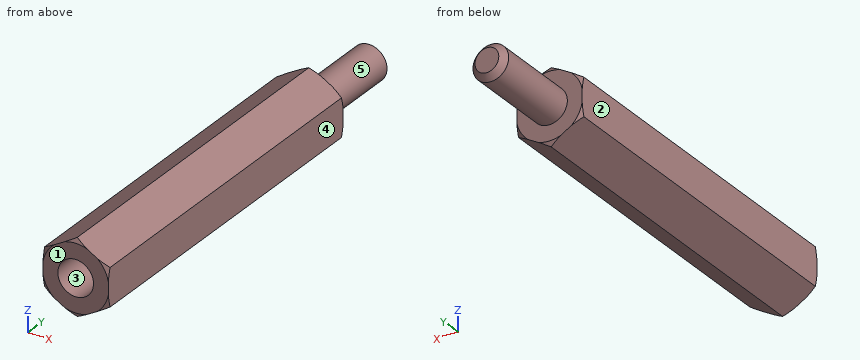
from build123d import *

# Parameters (mm, degrees)
SKETCH_1_R          = 1.5
EXTRUDE_1_DEPTH     = 30
SKETCH_3_R          = 1.5
EXTRUDE_2_DEPTH     = 8
CHAMFER_1_SIZE      = 0.5
SKETCH_1_3_R        = 1.5
CUT_EXTRUDE_1_DEPTH = 8


with BuildPart() as part:
    # Sketch 1 → Extrude 1 (new body)
    # profile 1 of 2: a face of its own
    with BuildSketch(Plane(origin=(0, 0, 0), x_dir=(1, 0, 0), z_dir=(0, 1, 0))):
        Polygon((2.75, -1.58771324), (2.75, 1.58771324), (0, 3.175426481), (-2.75, 1.58771324), (-2.75, -1.58771324), (0, -3.175426481), align=None)
        Circle(SKETCH_1_R, mode=Mode.SUBTRACT)
    # profile 2 of 2: a face of its own
    with BuildSketch(Plane(origin=(0, 0, 0), x_dir=(1, 0, 0), z_dir=(0, 1, 0))):
        Circle(SKETCH_1_R)
    extrude(amount=EXTRUDE_1_DEPTH)

    # Sketch 2 → Cut-Revolve 1 (revolve, cut)
    with BuildSketch(Plane(origin=(0, 0, 0), x_dir=(0, 0, -1), z_dir=(1, 0, 0))):
        Polygon((-26.160719749, 13.487317835), (-26.160719749, 0), (-2.8, 0), align=None)
        Polygon((-26.160719749, 30), (-26.160719749, 16.512682165), (-2.8, 30), align=None)
    revolve(axis=Axis((0, 30, 0), (0, -1, 0)), mode=Mode.SUBTRACT)

    # Sketch 3 → Extrude 2 (add)
    with BuildSketch(Plane(origin=(0, 30, 0), x_dir=(1, 0, 0), z_dir=(0, 1, 0))):
        with Locations(Location((0, 0, 0), (0, 0, 270))):
            Circle(SKETCH_3_R)
    extrude(amount=EXTRUDE_2_DEPTH)

    # Chamfer 1
    chamfer_1_edges = [part.edges().sort_by_distance(p)[0] for p in [
        (0, 38, -1.5),
    ]]
    chamfer(chamfer_1_edges, length=CHAMFER_1_SIZE)

    # Sketch 1_3 → Cut-Extrude 1 (cut)
    with BuildSketch(Plane(origin=(0, 0, 0), x_dir=(1, 0, 0), z_dir=(0, 1, 0))):
        with Locations(Location((0, 0, 0), (0, 0, 270))):
            Circle(SKETCH_1_3_R)
    extrude(amount=CUT_EXTRUDE_1_DEPTH, mode=Mode.SUBTRACT)


solid = part.part
Work out the finished part from the listing and answer in its coordinate system (mm). Face numbers are marked on the shaded views. A direction names the side the tool comes from. Give positions to 0.01 mm unless a question says otherwise; leave off trailing zeros. Order: outer loops, then holes, each group sorted by start corner. A loop starts at its lowest first (then second) coordinate and runs counter-clockwise, first axis right, second up. Notation, with made-up numbers: (63.25, -27) -> (67.25, -27) arc R18 cw to (67.25, -13) -> close; hole circle Ø7 at (39.25, -13). An arc over 180 degrees is marked (long way). Answer as a JSON object with one key per item and string values. Group by question number.
1. Consider line 1 along X through (y, z) = (2.25, 0); line 2 along Y through (x, z) = (-0.65, 0); line 3 along Y through (x, z) = (-1.9, 1.75). Determine where each line is inside the solid, lowest interval first. Write a range as [from, to].
2. Section A-A on y = 3 is taken. Determine the outline of the cut face in (x, z), plus the area to 3 significant figures.
3. Section C-C on y = 12 is taken. Determine the outline of the cut face in (x, z).
4. A tool of negligible diameter and unlimited length cuts with its end or side. For the marked faces 4 and 5, from which of +Z, -Z, +X, -X, +Y, -Y can it reach the whole face along a straight path? Write none if from no direction.
5. Flat-ended cylindrical pins translate along their axes: pin 1 Ø1 at (y, z) = (32, 1.5) entering from +X; pin 2 Ø1 at (x, y) = (-1, 14.5) entering from +Z; pin 3 Ø1 at (x, z) = (2, 1) entering from +Y. Find the tip coordinate at first contact, or state that the pin passes through.
6. Section D-D on y = 35 is taken. Determine the outline of the cut face in (x, z), plus the area to 3 significant figures.
7. Section B-B on z = 0 is taken. Determine the outline of the cut face in (x, y), plus the area to 3 significant figures.
8. The mould has two halves that part along X. Classify the marked faces 1, 2 and 3: released by +X, released by -X, zero draft, split by the parting line, or undercut.
Result sheet:
{
 "1": {"line 1": "x = [-2.75, -1.5], [1.5, 2.75]", "line 2": "y = [8, 38]", "line 3": "y = [0, 30]"},
 "2": {"outline": "(-2.75, -1.59) -> (0, -3.18) -> (2.75, -1.59) -> (2.75, 1.59) -> (0, 3.18) -> (-2.75, 1.59) -> close; hole circle Ø3 at (0, 0)", "area": "19.1 mm^2"},
 "3": {"outline": "(-2.75, -1.59) -> (0, -3.18) -> (2.75, -1.59) -> (2.75, 1.59) -> (0, 3.18) -> (-2.75, 1.59) -> close"},
 "4": {"face 4": "+Z, -Z, +X, +Y, -Y", "face 5": "+Y"},
 "5": {"pin 1": "stops at x = 1.12", "pin 2": "stops at z = 2.89", "pin 3": "stops at y = 30"},
 "6": {"outline": "circle Ø3 at (0, 0)", "area": "7.07 mm^2"},
 "7": {"outline": "(-2.75, 0) -> (-1.5, 0) -> (-1.5, 8) -> (1.5, 8) -> (1.5, 0) -> (2.75, 0) -> (2.75, 30) -> (1.5, 30) -> (1.5, 37.5) -> (1, 38) -> (-1, 38) -> (-1.5, 37.5) -> (-1.5, 30) -> (-2.75, 30) -> close", "area": "165 mm^2"},
 "8": {"face 1": "zero draft", "face 2": "released by -X", "face 3": "undercut"}
}
